The listing builds one solid part. Answer for the finished solid, in the listing's coordinates (mm). A direction names the side the tool comes from. Coordinates: 2 decimals unless noted, no trailing zeros. Order: outer loops, then holes, each group sorted by start corner. A loop starts at its lowest first (then second) coordinate and runs counter-clockwise, first axis right, second up. Notation, with made-up numbers: (46.5, 66.25) -> (70.5, 66.25) arc R32 ccw to (70.5, 101.25) -> close; hole circle Ø10 at (33, -26.5). An arc over 180 degrees is marked (long way). One line per question, with ' | ' between items.
from build123d import *

# Parameters (mm, degrees)
SKETCH2_R                     = 1.5
SKETCH2_R_2                   = 2
BASE_FLANGE1_DEPTH            = 1.4
EDGE_FLANGE1_STRIP_W          = 8.6
EDGE_FLANGE1_STRIP_H          = 1.4
EDGE_FLANGE1_STRIP_CUT_DEPTH  = 119.624404155
EDGE_FLANGE1_RELIEF_W         = 9.3
EDGE_FLANGE1_RELIEF_H         = 0.7
EDGE_FLANGE1_RELIEF_CUT_DEPTH = 1.4
EDGE_FLANGE1_DEPTH            = 119.624404155
SKETCH17_R                    = 1
CUT_EXTRUDE1_DEPTH            = 1.4


# Sheet-metal steps are written as plain solids
with BuildPart() as part:
    # Sketch2 → Base-Flange1 (new body)
    with BuildSketch(Plane.XY):
        with BuildLine():
            Line((231.478213009, 167.923533188), (111.868451864, 169.7951924))
            ThreePointArc((111.868451864, 169.7951924), (110.877145651, 169.910310621), (109.928447229, 170.220006467))
            Line((109.928447229, 170.220006467), (90.352175795, 178.856771959))
            ThreePointArc((90.352175795, 178.856771959), (89.060059005, 179.68413768), (88.079658187, 180.864355486))
            Line((88.079658187, 180.864355486), (81.624256856, 191.654630499))
            ThreePointArc((81.624256856, 191.654630499), (83.137635743, 199.512444421), (91.115351923, 198.886665029))
            Line((91.115351923, 198.886665029), (104.374715918, 187.262186129))
            ThreePointArc((104.374715918, 187.262186129), (105.880179055, 186.353553036), (107.60711557, 186.022307468))
            Line((107.60711557, 186.022307468), (189.939055045, 184.972638911))
            ThreePointArc((189.939055045, 184.972638911), (191.144825453, 185.104402623), (192.283387705, 185.522636952))
            Line((192.283387705, 185.522636952), (216.658747604, 198.015961736))
            ThreePointArc((216.658747604, 198.015961736), (217.779120548, 198.429892832), (218.965699032, 198.5662966))
            Line((218.965699032, 198.5662966), (266.21359493, 198.317204861))
            ThreePointArc((266.21359493, 198.317204861), (271.61517707, 194.425420779), (269.70061588, 188.049095159))
            Line((269.70061588, 188.049095159), (233.952189626, 168.534253774))
            ThreePointArc((233.952189626, 168.534253774), (232.754760905, 168.068640994), (231.478213009, 167.923533188))
        make_face()
        with Locations((86.776445718, 194.736984451)):
            Circle(SKETCH2_R, mode=Mode.SUBTRACT)
        with Locations((91.568382251, 182.289296649)):
            Circle(SKETCH2_R_2, mode=Mode.SUBTRACT)
        with Locations((208.186382216, 183.518819995)):
            Circle(SKETCH2_R, mode=Mode.SUBTRACT)
        with Locations((232.122136742, 192.086173294)):
            Circle(SKETCH2_R, mode=Mode.SUBTRACT)
        with Locations((266.183352442, 192.580788532)):
            Circle(SKETCH2_R_2, mode=Mode.SUBTRACT)
    extrude(amount=-BASE_FLANGE1_DEPTH)

    # Edge-Flange1 strip (across the edge) → Edge-Flange1 strip cut (cut)
    with BuildSketch(Plane(origin=(231.478213009, 167.923533188, -1.4), x_dir=(0.015646131950223352, 0.9998775917856126, -3.4914813388431334e-15), z_dir=(-0.9998775917856126, 0.015646131950223352, 0))):
        with Locations((-2.8, -0.7)):
            Rectangle(EDGE_FLANGE1_STRIP_W, EDGE_FLANGE1_STRIP_H)
    extrude(amount=EDGE_FLANGE1_STRIP_CUT_DEPTH, mode=Mode.SUBTRACT)

    # Edge-Flange1 relief (on the sheet) → Edge-Flange1 relief cut (cut)
    with BuildSketch(Plane(origin=(231.501682207, 169.423349576, -1.4), x_dir=(0.015646131950223352, 0.9998775917856126, -6.982962677686267e-15), z_dir=(0, 0, -1))):
        with Locations((-3.95, 0.35)):
            Rectangle(EDGE_FLANGE1_RELIEF_W, EDGE_FLANGE1_RELIEF_H)
        with Locations((-3.95, -119.974404155)):
            Rectangle(EDGE_FLANGE1_RELIEF_W, EDGE_FLANGE1_RELIEF_H)
    extrude(amount=-EDGE_FLANGE1_RELIEF_CUT_DEPTH, mode=Mode.SUBTRACT)

    # Edge-Flange1 section (across the edge) → Edge-Flange1 (add)
    with BuildSketch(Plane(origin=(231.478213009, 167.923533188, -1.4), x_dir=(0.015646131950223352, 0.9998775917856126, -3.4914813388431334e-15), z_dir=(-0.9998775917856126, 0.015646131950223352, 0))):
        with BuildLine():
            Line((-1.4, 1.5), (-1.4, 9.6))
            Line((-1.4, 9.6), (0, 9.6))
            Line((0, 9.6), (0, 1.5))
            ThreePointArc((0, 1.5), (0.439339828, 0.439339828), (1.5, 0))
            Line((1.5, 0), (1.5, -1.4))
            ThreePointArc((1.5, -1.4), (-0.550609665, -0.550609665), (-1.4, 1.5))
        make_face()
    extrude(amount=EDGE_FLANGE1_DEPTH)

    # Mirror1: part across plane


with BuildPart() as part_1:
    add(part.part)
    add(part.part.mirror(Plane(origin=(231.456308425, 166.52370456, -11), x_dir=(1, 0, 0), z_dir=(0, 0, 1))))

    # Sketch17 → Cut-Extrude1 (cut)
    with BuildSketch(Plane(origin=(0, 0, -22), x_dir=(-1, 0, 0), z_dir=(0, 0, -1))):
        with Locations(Location((-245.401847545, 191.466522217, 0), (0, 0, 90))):
            Circle(SKETCH17_R)
        with Locations(Location((-245.26459516, 181.540767155, 0), (0, 0, 90))):
            Circle(SKETCH17_R)
    extrude(amount=-CUT_EXTRUDE1_DEPTH, mode=Mode.SUBTRACT)


solid = part_1.part
Item 1: Section A-A, the plane x = 99 is taken. Give the vertices of the cut face in (y, z).
Computed values:
outline: (175.04, -22) -> (191.97, -22) -> (191.97, -20.6) -> (175.04, -20.6) -> close; (175.04, -1.4) -> (191.97, -1.4) -> (191.97, 0) -> (175.04, 0) -> close
Item 2: Find the intervals of material crossed by L1, parallel to Z at x = 121.5, y = 184; L2, parallel to X at y = 181.5, z = -20.75; L3, parallel to Z at x = 245, y = 182, in increasing order.
Computed values:
L1: z = -22 to -20.6, -1.4 to 0 | L2: x = 87.7 to 89.73, 93.41 to 244.27, 246.26 to 257.7 | L3: z = -1.4 to 0
Item 3: Section C-C, the plane z = -16 is taken. Give the vertices of the cut face in (x, y).
Computed values:
outline: (111.85, 168.4) -> (231.46, 166.52) -> (231.48, 167.92) -> (111.87, 169.8) -> close
Item 4: For faces 1 (the face through (252.08, 178.43, -21.31)), 2 (the face through (97.65, 193.16, -0.69)), 3 (the face through (172.517, 169.274, -1.851)), determine the directions among +Z, -Z, +X, -X, +Y, -Y from which every point of the face is accessible in a straight line to the end or side of a thin tool.
Computed values:
face 1: +Z, -Z, +X, -Y | face 2: +Z, -Z, +Y | face 3: +X, +Y
Item 5: Section B-B, the plane y = 175 is taken. Give the vertices of the cut face in (x, z), plus the area to 3 significant figures.
Computed values:
outline: (99.09, -22) -> (245.8, -22) -> (245.8, -20.6) -> (99.09, -20.6) -> close; (99.09, -1.4) -> (245.8, -1.4) -> (245.8, 0) -> (99.09, 0) -> close | area: 411 mm^2
Item 6: Each of these flat-tipped pins is pushed along its axis until it touches: pin 1 Ø1.5 at (x, z) = (223.5, -18.5) entering from +Y; pin 2 Ø1.2 at (x, y) = (245.4, 191.47) entering from -Z; pin 3 Ø1 at (x, z) = (144.5, -15) entering from +Y. Where does it stop, or does it pass through?
Computed values:
pin 1: stops at y = 168.06 | pin 2: stops at z = -1.4 | pin 3: stops at y = 169.29
Item 7: Determine the mould class of faces 4 (the face through (178, 181, -22)), 5 (the face through (264.6, 191.36, -21.31)), 6 (the face through (97.65, 193.16, -21.31)) for opening direction Y: pulls with the +Y half, pulls with the -Y half, needs draft (parallel to the pull), parting line crosses it, or undercut.
Computed values:
face 4: needs draft | face 5: undercut | face 6: pulls with the +Y half
